The listing builds one solid part. Answer for the finished solid, in the listing's coordinates (mm). Round coordinates to 2 decimals unless told otherwise and drop trailing zeros. Write each loop counter-clockwise with the first axis right and the second up, starting at its lowest first coordinate (ties: lowest second). Pieces come first, ordered by that corner, then holes.
Item 1: Find the intervals of material crossed by probe 1 along Y at (x, z) = (-36.5, -7.25); probe 2 along Y at (x, z) = (3.5, -1.75), in increasing order.
Item 2: Each of these flat-tipped pins is pushed along its axis until it touches: pin 1 (1.8 mm diameter, centred on x = -56.87, y = 5.73, fed in from -Z); pin 2 (3.5 mm diameter, centred on x = -16.23, y = 5.73, fed in from -Z). Where does it stop, or does it pass through?
Item 3: Find section A-A on x = -16.5. Give the vertices of the cut face in (y, z).
```python
from build123d import *

# Parameters (mm, degrees)
F0_W     = 71.0019436256
F0_H     = 25.4
F0_R     = 1.016
F1_DEPTH = 12.7
F2_R     = 0.508


# Not quite as in the source:
# - a feature names something its author has since deleted; it is built from what else it names


with BuildPart() as f1:
    # F0 (on Top) → F1 (new body)
    with BuildSketch(Plane.XY):
        with Locations((-26.4490794038, 5.7338142046)):
            Rectangle(F0_W, F0_H)
        with Locations((-56.8700512166, 5.7338142046)):
            Circle(F0_R, mode=Mode.SUBTRACT)
        with Locations((-46.7100512166, 5.7338142046)):
            Circle(F0_R, mode=Mode.SUBTRACT)
        with Locations((-36.5500512166, 5.7338142046)):
            Circle(F0_R, mode=Mode.SUBTRACT)
        with Locations((-26.3900512166, 5.7338142046)):
            Circle(F0_R, mode=Mode.SUBTRACT)
        with Locations((-16.2300512166, 5.7338142046)):
            Circle(F0_R, mode=Mode.SUBTRACT)
        with Locations((-6.0700512166, 5.7338142046)):
            Circle(F0_R, mode=Mode.SUBTRACT)
        with Locations((4.0899487834, 5.7338142046)):
            Circle(F0_R, mode=Mode.SUBTRACT)
    extrude(amount=-F1_DEPTH)

    # F2
    f2_edges = [f1.edges().sort_by_distance(p)[0] for p in [
        (-26.449079, 18.433814, 0),
        (-26.449079, -6.966186, 0),
        (-61.950051, 5.733814, 0),
        (-61.950051, -6.966186, -6.35),
        (-61.950051, 18.433814, -6.35),
        (-26.449079, 18.433814, -12.7),
        (-61.950051, 5.733814, -12.7),
        (-26.449079, -6.966186, -12.7),
        (9.051892, 5.733814, -12.7),
        (9.051892, 5.733814, 0),
        (9.051892, 18.433814, -6.35),
        (9.051892, -6.966186, -6.35),
    ]]
    fillet(f2_edges, radius=F2_R)


solid = f1.part
```
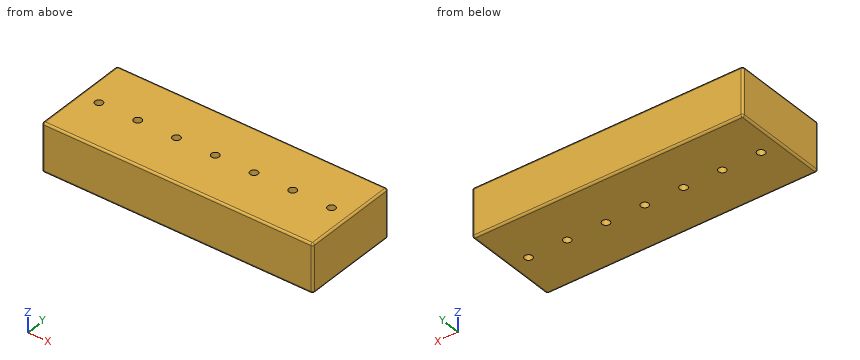
Check values:
1. probe 1: y = -6.97 to 4.72, 6.75 to 18.43
1. probe 2: y = -6.97 to 4.91, 6.56 to 18.43
2. pin 1: passes through
2. pin 2: stops at z = -12.7
3. outline: (-6.97, -12.19) arc R0.51 ccw to (-6.46, -12.7) - (4.75, -12.7) - (4.75, 0) - (-6.46, 0) arc R0.51 ccw to (-6.97, -0.51) - close; (6.71, -12.7) - (17.93, -12.7) arc R0.51 ccw to (18.43, -12.19) - (18.43, -0.51) arc R0.51 ccw to (17.93, 0) - (6.71, 0) - close
